For this review, take the finished solid that the model builds, in its own axes (mm). A direction names the side the tool comes from. Round coordinates to 2 decimals unless told otherwise and drop trailing zeros. Write each loop counter-clockwise with the first axis right and the second up, starting at its lowest first coordinate (ties: lowest second). Pieces come first, ordered by that corner, then holes. Notation, with made-up numbers: M 29,-30.5 L 86,-30.5 A21 cw 86,-12.5 Z; hole C 11,-25.5 d7. An arc over 180 degrees is marked long. Use one line per item in the form item = value. Start each with the question number.
Item 1: Add section A-A (x = 43). State the section outline as (y, z) points, and give its area (3 significant figures).
Item 2: Add section B-B (z = 31). State the section outline as (x, y) points.
Item 3: For line 1 (Z direction, x = 29, y = 17); line 2 (Z direction, x = 41.5, y = 4); line 3 (Z direction, x = 44.5, y = -44), list the stretches that pass through material, from the lowest coordinate up. Write a range as [from, to].
Item 4: For P1, Ø8, axis at y = 9, z = 51.5, coming from the -X side; P2, Ø10, axis at x = 6, z = 33, coming from the +Y side; P3, Ø6, axis at x = 16.5, y = 15.5, coming from the +Z side, all flat-tipped, find the tip position at first contact; note any pin that passes through.
Item 5: Add section C-C (y = -19). State the section outline as (x, z) points.
Item 6: For faces 5 (the flat face through (35, 10, 43.5)), 6 (the flat face through (35, 10, 42)), 7 (the flat face through (25, 10, 43)), list the 3-axis set-ups (+Z, -Z, +X, -X, +Y, -Y) from which the entire face can be reached by the end or side of a thin tool; tool diameter is ignored.
Item 7: Draft analysis for pull direction Y (two halves, no side actions). For faces 1 (the flat face through (48, 50, 28)), 2 (the flat face through (35, 16.5, 50)), 3 (the flat face through (35, 2, 50)), 4 (the flat face through (-3, 3, 5)), state which applies: released by +Y, released by -Y, zero draft, split by the parting line, or undercut.
from build123d import *

# Parameters (mm, degrees)
SKETCH1_W           = 100
SKETCH1_H           = 100
BOSS_EXTRUDE1_DEPTH = 5
BOSS_EXTRUDE4_DEPTH = 95
SKETCH5_W           = 16
SKETCH5_H           = 16
BOSS_EXTRUDE6_DEPTH = 20
SKETCH8_W           = 13
SKETCH8_H           = 13
CUT_EXTRUDE2_DEPTH  = 20
SKETCH9_R           = 2
CUT_EXTRUDE3_DEPTH  = 5


with BuildPart() as part:
    # Sketch1 → Boss-Extrude1 (new body)
    with BuildSketch(Plane.XY):
        Rectangle(SKETCH1_W, SKETCH1_H)
    extrude(amount=BOSS_EXTRUDE1_DEPTH)

    # Sketch4 → Boss-Extrude4 (add)
    with BuildSketch(Plane.XY.offset(5)):
        Polygon((50, 50), (50, -50), (-50, -50), (-50, -45), (45, -45), (45, 50), align=None)
    extrude(amount=BOSS_EXTRUDE4_DEPTH)

    # Sketch5 → Boss-Extrude6 (add)
    with BuildSketch(Plane.ZY.offset(-45)):
        with Locations((50, 10)):
            Rectangle(SKETCH5_W, SKETCH5_H)
    extrude(amount=BOSS_EXTRUDE6_DEPTH)

    # Sketch8 → Cut-Extrude2 (cut)
    with BuildSketch(Plane.ZY.offset(-25)):
        with Locations((50, 10)):
            Rectangle(SKETCH8_W, SKETCH8_H)
    extrude(amount=-CUT_EXTRUDE2_DEPTH, mode=Mode.SUBTRACT)

    # Sketch9 → Cut-Extrude3 (cut)
    with BuildSketch(Plane(origin=(0, 18, 0), x_dir=(1, 0, 0), z_dir=(0, 1, 0))):
        with Locations(Location((39.3, -49.816402155, 0), (0, 0, 180))):
            Circle(SKETCH9_R)
        with Locations(Location((29.3, -49.816402155, 0), (0, 0, 180))):
            Circle(SKETCH9_R)
    extrude(amount=-CUT_EXTRUDE3_DEPTH, mode=Mode.SUBTRACT)


solid = part.part
Calculated:
q1.outline = M -50,0 L 50,0 L 50,5 L -45,5 L -45,100 L -50,100 Z; M 2,42 L 18,42 L 18,58 L 2,58 Z; hole M 3.5,43.5 L 16.5,43.5 L 16.5,56.5 L 3.5,56.5 Z
q1.area = 1,060 mm^2
q2.outline = M -50,-50 L 50,-50 L 50,50 L 45,50 L 45,-45 L -50,-45 Z
q3.line_1 = [0, 5], [42, 47.84], [51.79, 58]
q3.line_2 = [0, 5], [42, 43.5], [56.5, 58]
q3.line_3 = [0, 5]
q4.P1 = 45
q4.P2 = -45
q4.P3 = 5
q5.outline = M -50,0 L 50,0 L 50,100 L 45,100 L 45,5 L -50,5 Z
q6.face_5 = -X
q6.face_6 = -X, +Y
q6.face_7 = +Z, -X, +Y
q7.face_1 = released by +Y
q7.face_2 = undercut
q7.face_3 = undercut
q7.face_4 = zero draft
